Here's how the part is built. I have some questions about the finished solid (model axes, mm). Face numbers are marked on the shaded views. A direction names the side the tool comes from. Give positions to 0.01 mm unless a question says otherwise; leave off trailing zeros. Loops run counter-clockwise (first coordinate to the right, second up) from the corner with the lowest first, then second, coordinate; pieces in that order, holes last.
Q1. I need wall thicknesses on line 1 (X direction, y = -37.5, z = 0.5); line 2 (X direction, y = -66, z = 2.5); line 3 (Y direction, x = -18, z = 5.25). Which ranges of each line are inside material? Lowest first, please.
Q2. If we section it at D-D (y = -64): Give the number of separate pieces and of enclosed holes in the cut face, plus the area to 3 significant figures.
Q3. If we section it at A-A (x = 10): Please give me the cut outline in (y, z), plus the area to 3 significant figures.
Q4. If we section it at C-C (y = 25): Please give me the cut outline in (x, z) (3 decimals), plus the area to 3 significant figures.
Q5. If we section it at B-B (y = -41.5): Please give me the cut outline in (x, z).
Q6. Will this pin go through, and if not, where does the flat tip stop? P1, Ø4, axis at x = 10, y = -25, coming from the -Z side.
Q7. For the marked faces 1 and 2, which set-ups out of +Z, -Z, +X, -X, +Y, -Y let a thin tool reach every point of the face, with its end or its side?
Q8. We'd pull the mould along X, two halves only. Please class the marked faces 3, 4 and 5: +X half, -X half, draft (parallel to the pull), parting line (faces both ways), or undercut.
Autodesk Inventor part; units mm, degrees
ref_plane "YZ Plane" through (0, 0, 0) normal (1, 0, 0) x (0, 1, 0)
ref_plane "XZ Plane" through (0, 0, 0) normal (0, 1, 0) x (-1, 0, 0)
ref_plane "XY Plane" through (0, 0, 0) normal (0, 0, 1) x (1, 0, 0)
ref_plane "Work Plane1" through (0, 0, 0) normal (0, 0, 1) x (1, 0, 0)
sketch "Sketch1" plane through (0, 0, 0) normal (0, 0, 1) x (1, 0, 0)
  circle A0 centre (-10, -25) radius 1.45
  circle A1 centre (-10, 25) radius 1.45
  circle A2 centre (10, 25) radius 1.45
  circle A3 centre (10, -25) radius 1.45
  circle A4 centre (-25, 25) radius 2.325
  circle A5 centre (25, -25) radius 2.325
  circle A6 centre (-25, -25) radius 2.325
  circle A7 centre (25, 25) radius 2.325
  line L0 (28, 30) -> (30, 28)
  line L1 (28, 30) -> (-28, 30)
  line L2 (-30, 28) -> (-28, 30)
  line L3 (-30, 28) -> (-30, -28)
  line L4 (-28, -30) -> (-30, -28)
  line L5 (-28, -30) -> (28, -30)
  line L6 (30, -28) -> (28, -30)
  line L7 (30, -28) -> (30, 28)
  circle A8 centre (-17.5, -17.5) radius 1.95
  circle A9 centre (17.5, 17.5) radius 1.95
  circle A10 centre (17.5, -17.5) radius 1.95
  circle A11 centre (-17.5, 17.5) radius 1.95
  circle A12 centre (0, 0) radius 7.5
  circle A13 centre (-25.33, -75.26) radius 6.15
  circle A14 centre (25, -10) radius 1.45
  circle A15 centre (-25, -10) radius 1.45
  circle A16 centre (-25, 10) radius 1.45
  circle A17 centre (25, 10) radius 1.45
  point P0 (0, 0)
extrude "Extrusion1" add sketch "Sketch1" along normal blind 8 contours L0 L7 L6 L5 L4 L3 L2 L1
sketch "Sketch2" plane through (0, 0, 8) normal (0, 0, 1) x (1, 0, 0)
  circle A0 centre (0, 0) radius 7.5
  circle A1 centre (25, 10) radius 1.45
  circle A2 centre (-25, 10) radius 1.45
  circle A3 centre (-25, -10) radius 1.45
  circle A4 centre (25, -10) radius 1.45
  circle A5 centre (10, -25) radius 1.45
  circle A6 centre (10, 25) radius 1.45
  circle A7 centre (-10, 25) radius 1.45
  circle A8 centre (-10, -25) radius 1.45
  line L0 (-28, -30) -> (28, -30)
  line L1 (28, -30) -> (30, -28)
  line L2 (30, -28) -> (30, 28)
  line L3 (30, 28) -> (28, 30)
  line L4 (28, 30) -> (-28, 30)
  line L5 (30, -28) -> (30, 28)
  line L6 (30, -30) -> (16, -30)
  line L7 (16, -30) -> (16, -80)
  line L8 (16, -80) -> (30, -80)
  line L9 (30, -80) -> (30, -30)
  line L10 (30, 28) -> (30, -28)
  line L11 (30, -30) -> (30, -28)
  line L12 (30, -28) -> (28, -30)
  line L13 (-28, 30) -> (-30, 28)
  line L14 (-30, 28) -> (-30, -28)
  line L15 (-30, -28) -> (-28, -30)
  line L16 (-30, -30) -> (-14, -30)
  line L17 (-14, -30) -> (-14, -80)
  line L18 (-14, -80) -> (-30, -80)
  line L19 (-30, -80) -> (-30, -30)
  line L20 (-30, -30) -> (-30, -28)
  line L21 (-30, -28) -> (-28, -30)
  line L22 (-28, -30) -> (-30, -30)
  line L23 (28, -30) -> (30, -28)
  line L24 (28, -30) -> (30, -30)
  line L25 (30, -30) -> (30, -28)
  line L26 (30, -28) -> (28, -30)
  circle A9 centre (-17.5, 17.5) radius 1.95
  circle A10 centre (-25, 25) radius 2.325
  circle A11 centre (25, 25) radius 2.325
  circle A12 centre (17.5, 17.5) radius 1.95
  circle A13 centre (17.5, -17.5) radius 1.95
  circle A14 centre (25, -25) radius 2.325
  circle A15 centre (-25, -25) radius 2.325
  point P0 (0, 0)
  point P1 (-24.2387, -104)
  dimension "d57" = 14
  dimension "d58" = 50
  dimension "d59" = 16
extrude "Extrusion2" add sketch "Sketch2" against normal up to surface (8 mm away) contours L16 L20 L15 | L0 L17 L18 L19 L16 | L0 L6 L9 L8 L7 | L1 L11 L6
fillet "Fillet1" radius 4 6 edges at (30, -80, 4) (16, -80, 4) (-14, -80, 4) (-30, -80, 4) (-14, -30, 4) (16, -30, 4)
ref_plane "Work Plane2" through (-6, -91, 19) normal (1, 0, 0) x (0, 0, -1)
sketch "Sketch8" plane through (0, 0, 8) normal (0, 0, 1) x (1, 0, 0)
  circle A0 centre (0, 0) radius 16
  point P0 (0, 0)
  dimension "d41" = 32
extrude "Extrusion7" cut sketch "Sketch8" against normal through all
sketch "Sketch11" plane through (0, 0, 8) normal (0, 0, 1) x (1, 0, 0)
  circle A0 centre (0, 0) radius 16
  circle A1 centre (25, 25) radius 2.325
  circle A2 centre (-25, -25) radius 2.325
  circle A3 centre (25, -25) radius 2.325
  circle A4 centre (-25, 25) radius 2.325
  circle A5 centre (-17.5, 17.5) radius 1.95
  circle A6 centre (17.5, -17.5) radius 1.95
  circle A7 centre (17.5, 17.5) radius 1.95
  circle A8 centre (-17.5, -17.5) radius 1.95
  circle A9 centre (25, 10) radius 1.45
  circle A10 centre (-25, 10) radius 1.45
  circle A11 centre (-25, -10) radius 1.45
  circle A12 centre (25, -10) radius 1.45
  circle A13 centre (10, -25) radius 1.45
  circle A14 centre (10, 25) radius 1.45
  circle A15 centre (-10, 25) radius 1.45
  circle A16 centre (-10, -25) radius 1.45
  arc A17 (16, -76) -> (20, -80) centre (20, -76) ccw
  line L0 (20, -80) -> (26, -80)
  arc A18 (26, -80) -> (30, -76) centre (26, -76) ccw
  line L1 (30, 28) -> (30, -76)
  line L2 (30, 28) -> (28, 30)
  line L3 (28, 30) -> (-28, 30)
  line L4 (-28, 30) -> (-30, 28)
  line L5 (-10, -30) -> (12, -30)
  arc A19 (16, -34) -> (12, -30) centre (12, -34) ccw
  line L6 (16, -34) -> (16, -76)
  circle A20 centre (23, -74) radius 3.75
  circle A21 centre (23, -64) radius 1.45
  circle A22 centre (23, -54) radius 1.45
  arc A23 (-30, -76) -> (-26, -80) centre (-26, -76) ccw
  line L7 (-18, -80) -> (-26, -80)
  arc A24 (-18, -80) -> (-14, -76) centre (-18, -76) ccw
  line L8 (-14, -34) -> (-14, -76)
  arc A25 (-10, -30) -> (-14, -34) centre (-10, -34) ccw
  line L9 (-30, 28) -> (-30, -76)
  point P0 (0, 0)
  dimension "d77" = 7.5
  dimension "d80" = 2.9
  dimension "d81" = 2.9
  dimension "d82" = 10
  dimension "d83" = 10
  dimension "d84" = 6
extrude "Extrusion10" cut sketch "Sketch11" against normal through all contours A20 | A21 | A22
sketch "Sketch12" plane through (16, -76, 8) normal (-1, 0, 0) x (0, 0, 1)
  line L0 (-8, -1.75) -> (-8, 5.75)
  line L1 (0, 5.75) -> (0, -1.75)
  circle A0 centre (-4.3852, 2) radius 1.45
  point P0 (-8, 76)
  dimension "d85" = 2.9
extrude "Extrusion11" cut sketch "Sketch12" against normal through all
sketch "Sketch13" plane through (0, 0, 8) normal (0, 0, 1) x (1, 0, 0)
  circle A0 centre (23, -54) radius 1.45
  circle A1 centre (23, -64) radius 1.45
  circle A2 centre (23, -74) radius 3.75
  circle A3 centre (0, 0) radius 16
  arc A4 (-30, -76) -> (-26, -80) centre (-26, -76) ccw
  line L0 (-30, -76) -> (-30, 28)
  line L1 (-30, 28) -> (-28, 30)
  line L2 (-28, 30) -> (28, 30)
  line L3 (28, 30) -> (30, 28)
  line L4 (30, 28) -> (30, -76)
  arc A5 (26, -80) -> (30, -76) centre (26, -76) ccw
  line L5 (26, -80) -> (20, -80)
  arc A6 (16, -76) -> (20, -80) centre (20, -76) ccw
  line L6 (16, -76) -> (16, -34)
  arc A7 (16, -34) -> (12, -30) centre (12, -34) ccw
  line L7 (12, -30) -> (-10, -30)
  arc A8 (-10, -30) -> (-14, -34) centre (-10, -34) ccw
  line L8 (-14, -34) -> (-14, -76)
  arc A9 (-18, -80) -> (-14, -76) centre (-18, -76) ccw
  line L9 (-18, -80) -> (-26, -80)
  circle A10 centre (25, 25) radius 2.325
  circle A11 centre (-25, -25) radius 2.325
  circle A12 centre (25, -25) radius 2.325
  circle A13 centre (-25, 25) radius 2.325
  circle A14 centre (-17.5, 17.5) radius 1.95
  circle A15 centre (17.5, -17.5) radius 1.95
  circle A16 centre (17.5, 17.5) radius 1.95
  circle A17 centre (-17.5, -17.5) radius 1.95
  circle A18 centre (25, 10) radius 1.45
  circle A19 centre (-25, 10) radius 1.45
  circle A20 centre (-25, -10) radius 1.45
  circle A21 centre (25, -10) radius 1.45
  circle A22 centre (10, -25) radius 1.45
  circle A23 centre (10, 25) radius 1.45
  circle A24 centre (-10, 25) radius 1.45
  circle A25 centre (-10, -25) radius 1.45
  line L10 (-36.3192, -79.6068) -> (-18.6416, -61.9292)
  line L11 (-18.6416, -61.9292) -> (-17.5809, -62.9898)
  line L12 (-17.5809, -62.9898) -> (-35.2586, -80.6675)
  line L13 (-35.2586, -80.6675) -> (-36.3192, -79.6068)
  line L14 (-36.3192, -79.6068) -> (-17.5809, -62.9898) construction
  line L15 (-18.6416, -61.9292) -> (-35.2586, -80.6675) construction
  line L16 (-36.3192, -79.6068) -> (-11.3192, -79.6068) construction
  point P0 (0, 0)
  point P1 (-26.9501, -71.2983)
  dimension "d88" = 25
  dimension "d89" = 45
  dimension "d90" = 1.5
extrude "Extrusion12" cut sketch "Sketch13" against normal blind 10 contours L12 L13 L10 L0 | L0 L10 L11 L12
sketch "Sketch14" plane through (-15.0607, -58.3483, 8) normal (-0.7071, 0.7071, 0) x (-0.7071, -0.7071, 0)
  line L0 (22.6274, -8) -> (5.0642, -8)
  line L1 (5.0642, 0) -> (22.6274, 0)
  line L2 (5.0642, 0) -> (5.0642, -8)
  circle A0 centre (18.1437, -4) radius 1.45
  circle A1 centre (10.5109, -4) radius 1.45
  line L3 (22.6274, 0) -> (22.6274, -8)
  point P0 (-51.9079, -8)
  dimension "d93" = 2.9
  dimension "d94" = 2.9
extrude "Extrusion13" cut sketch "Sketch14" along normal through all contours A0 | A1
ref_plane "Work Plane3" through (0, 28, 0) normal (-1, 0, 0) x (0, 0, 1)
properties part number "30_XY_Sample_lightsheetarm_v3"
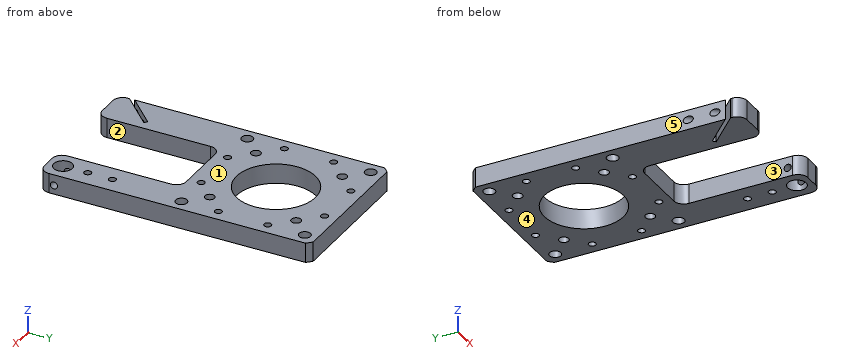
Check sheet entries:
1. line 1: x = -30 to -14, 16 to 30
1. line 2: x = -30 to -22.71, -20.59 to -14, 16 to 30
1. line 3: y = -80 to -63.41, -62.57 to -19.38, -15.62 to 15.62, 19.38 to 30
2. separate pieces: 4
2. enclosed holes: 1
2. area: 190 mm2
3. outline: (-30, 0) - (-26.45, 0) - (-26.45, 8) - (-30, 8) - close; (-23.55, 0) - (-12.49, 0) - (-12.49, 8) - (-23.55, 8) - close; (12.49, 0) - (23.55, 0) - (23.55, 8) - (12.49, 8) - close; (26.45, 0) - (30, 0) - (30, 8) - (26.45, 8) - close
3. area: 234 mm2
4. outline: (-30, 0) - (-27.325, 0) - (-27.325, 8) - (-30, 8) - close; (-22.675, 0) - (-11.45, 0) - (-11.45, 8) - (-22.675, 8) - close; (-8.55, 0) - (8.55, 0) - (8.55, 8) - (-8.55, 8) - close; (11.45, 0) - (22.675, 0) - (22.675, 8) - (11.45, 8) - close; (27.325, 0) - (30, 0) - (30, 8) - (27.325, 8) - close
4. area: 359 mm2
5. outline: (-30, 0) - (-14, 0) - (-14, 8) - (-30, 8) - close; (16, 0) - (30, 0) - (30, 8) - (16, 8) - close
6. P1: stops at z = 0
7. face 1: +Z, +X, -X, +Y, -Y
7. face 2: +Z, -Z, -Y
8. face 3: undercut
8. face 4: draft
8. face 5: -X half
